Check sheet for the modelled part. Datum: model origin and axes. Units: mm. A direction names the side the tool comes from. Give positions to 0.01 mm unless a question says otherwise; leave off trailing zeros. Order: outer loops, then holes, each group sorted by start corner. A loop starts at its lowest first (then second) coordinate and runs counter-clockwise, first axis right, second up. Notation, with made-up numbers: (36, -1.75) -> (41, -1.75) arc R5 ccw to (41, 3.25) -> close; hole circle Ø10 at (-7.75, 40). An arc over 180 degrees is marked (long way). Answer in a Markdown table with one row per item. Add a question column.
(1) Thickness scan on L1, parallel to X at y = 0, z = 22; L2, parallel to X at y = 0, z = 26; L3, parallel to Z at x = -22, y = 48. Record the ranges inside material, lowest first. Write a range as [from, to].
(2) Go/stop test with flat-tipped pins: pin 1 (8 mm diameter, centred on y = 9.5, z = 43.5, fed in from -X); pin 2 (1 mm diameter, centred on x = -34.5, y = -37, fed in from +Z); pin 3 (12 mm diameter, centred on x = -24, y = 11, fed in from -Z). Record where each tip stops, or that it passes through.
(3) Release check for a two-part mould opening along X. For faces 1 (the face through (-18, -59.231, 13)), 2 (the face through (-24.846, -22.617, 25.044)), 3 (the face through (-42.13, -17.47, 37.92)), 4 (the face through (18.868, 0, 13)) record: released by +X, released by -X, zero draft, split by the parting line, or undercut.
(4) Cross-section at A-A (y = 0). Record the cut outline in (x, z), then the cut area to 3 significant figures.
(5) Cross-section at C-C (x = -35). Record the cut outline in (y, z).
(6) Set-up check for faces 5 (the face through (-10, 28, 25.4)), 6 (the face through (-54.216, 0, 13)): record each of +Z, -Z, +X, -X, +Y, -Y from which the full face is reachable in a straight line by a thin tool's end or side.
(7) Cross-section at D-D (y = -40). Record the cut outline in (x, z), then the cut area to 3 significant figures.
(8) Cross-section at B-B (z = 4.5). Record the cut outline in (x, y), then the cut area to 3 significant figures.
```python
from build123d import *

# Parameters (mm, degrees)
F1_R     = 28.7120004049
F2_DEPTH = 50.8
F0_W     = 73.0837620795
F0_H     = 120.1344206929
F3_DEPTH = 25.4
F4_R     = 23.1683066689
F5_DEPTH = 149.098
F6_DEPTH = 50.8


with BuildPart() as f2:
    # F1 (on Top) → F2 (new body)
    with BuildSketch(Plane.XY):
        with Locations((-19.3457026035, 0)):
            Circle(F1_R)
    extrude(amount=F2_DEPTH)

    # F0 (on Top) → F3 (join)
    with BuildSketch(Plane.XY):
        with Locations((-17.6738519222, 0.8359253407)):
            Rectangle(F0_W, F0_H)
    extrude(amount=F3_DEPTH)

    # F4 (on Top) → F5 (cut)
    with BuildSketch(Plane.XY):
        with Locations((-19.8233742267, 0)):
            Circle(F4_R)
    extrude(amount=F5_DEPTH, mode=Mode.SUBTRACT)

    # F4 (on Top) → F6 (cut)
    with BuildSketch(Plane.XY):
        with Locations((-19.8233742267, 0)):
            Circle(F4_R)
    extrude(amount=F6_DEPTH, mode=Mode.SUBTRACT)


solid = f2.part
```
Answer below:
| question | item | result |
|---|---|---|
| 1 | L1 | x = [-54.22, -42.99], [3.34, 18.87] |
| 1 | L2 | x = [-48.06, -42.99], [3.34, 9.37] |
| 1 | L3 | z = [0, 25.4] |
| 2 | pin 1 | stops at x = -47.53 |
| 2 | pin 2 | stops at z = 25.4 |
| 2 | pin 3 | passes through |
| 3 | face 1 | zero draft |
| 3 | face 2 | undercut |
| 3 | face 3 | split by the parting line |
| 3 | face 4 | released by +X |
| 4 | outline | (-54.22, 0) -> (-42.99, 0) -> (-42.99, 50.8) -> (-48.06, 50.8) -> (-48.06, 25.4) -> (-54.22, 25.4) -> close; (3.34, 0) -> (18.87, 0) -> (18.87, 25.4) -> (9.37, 25.4) -> (9.37, 50.8) -> (3.34, 50.8) -> close |
| 4 | area | 961 mm² |
| 5 | outline | (-59.23, 0) -> (-17.51, 0) -> (-17.51, 50.8) -> (-24.07, 50.8) -> (-24.07, 25.4) -> (-59.23, 25.4) -> close; (17.51, 0) -> (60.9, 0) -> (60.9, 25.4) -> (24.07, 25.4) -> (24.07, 50.8) -> (17.51, 50.8) -> close |
| 6 | face 5 | +Z |
| 6 | face 6 | +Z, -Z, -X, +Y, -Y |
| 7 | outline | (-54.22, 0) -> (18.87, 0) -> (18.87, 25.4) -> (-54.22, 25.4) -> close |
| 7 | area | 1,860 mm² |
| 8 | outline | (-54.22, -59.23) -> (18.87, -59.23) -> (18.87, 60.9) -> (-54.22, 60.9) -> close; hole circle Ø46.34 at (-19.82, 0) |
| 8 | area | 7,090 mm² |
